```python
from build123d import *

# Parameters (mm, degrees)
SKETCH_1_R              = 4.25
EXTRUDE_1_DEPTH         = 1
SKETCH_2_R              = 3.5
EXTRUDE_2_DEPTH         = 10
HOLE_WIZARD_M31_D       = 3.4
HOLE_WIZARD_M31_DEPTH   = 5
HOLE_WIZARD_M31_TIP     = 1.021463052
CHAMFER_1_SIZE          = 0.5
HOLE_WIZARD_M31_2_D     = 2.5
HOLE_WIZARD_M31_2_DEPTH = 3
HOLE_WIZARD_M31_2_TIP   = 0.751075774


with BuildPart() as part:
    # Эскиз1 → Бобышка-Вытянуть1 (new body)
    with BuildSketch(Plane.XY):
        Circle(SKETCH_1_R)
    extrude(amount=EXTRUDE_1_DEPTH)

    # Эскиз2 → Бобышка-Вытянуть2 (add)
    with BuildSketch(Plane.XY.offset(1)):
        Circle(SKETCH_2_R)
    extrude(amount=EXTRUDE_2_DEPTH)

    # Hole Wizard M31
    with Locations(Plane.XY.offset(11)):
        with Locations((0, 0)):
            Hole(HOLE_WIZARD_M31_D / 2, depth=HOLE_WIZARD_M31_DEPTH)
            with Locations((0, 0, -(HOLE_WIZARD_M31_DEPTH + HOLE_WIZARD_M31_TIP / 2))):  # 118° drill point
                Cone(0, HOLE_WIZARD_M31_D / 2, HOLE_WIZARD_M31_TIP, mode=Mode.SUBTRACT)

    # Фаска1
    chamfer_1_edges = [part.edges().sort_by_distance(p)[0] for p in [
        (1.7, 0, 11),
    ]]
    chamfer(chamfer_1_edges, length=CHAMFER_1_SIZE)

    # Hole Wizard M31 2
    with Locations(Plane(origin=(0.206904612, 3.493879002, 8), x_dir=(0.998251143468, -0.059115603402, 0), z_dir=(0.059115603402, 0.998251143468, 0))):
        with Locations((0, 0)):
            Hole(HOLE_WIZARD_M31_2_D / 2, depth=HOLE_WIZARD_M31_2_DEPTH)
            with Locations((0, 0, -(HOLE_WIZARD_M31_2_DEPTH + HOLE_WIZARD_M31_2_TIP / 2))):  # 118° drill point
                Cone(0, HOLE_WIZARD_M31_2_D / 2, HOLE_WIZARD_M31_2_TIP, mode=Mode.SUBTRACT)


solid = part.part
```
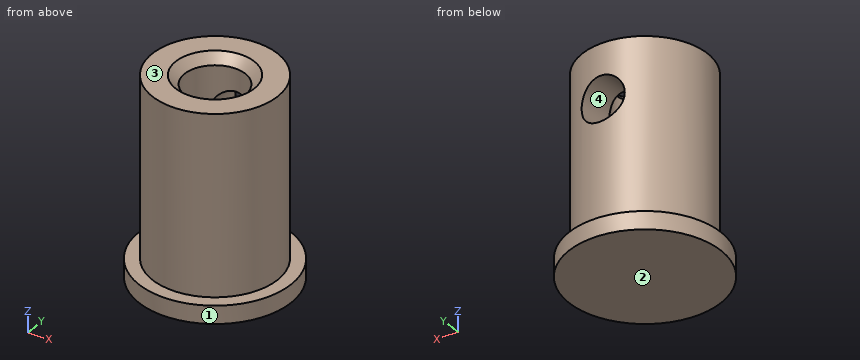
Here's how the part is built. I have some questions about the finished solid (model axes, mm). Face numbers are marked on the shaded views. Round coordinates to 2 decimals unless told otherwise and drop trailing zeros. Loops run counter-clockwise (first coordinate to the right, second up) from the corner with the lowest first, then second, coordinate; pieces in that order, holes last.
1. Will these pins go through, and if not, where does the flat tip stop? pin 1 (4 mm diameter, centred on y = 3, z = 2.5, fed in from +X); pin 2 (5 mm diameter, centred on y = 2.5, z = 9, fed in from -X).
Answers:
pin 1: stops at x = 3.91
pin 2: stops at x = -3.5
2. Suppose I cut it at C-C, the plane y = -3. Please give me the cut outline in (x, z), and give its area (3 significant figures).
Answers:
outline: (-3.01, 0) - (3.01, 0) - (3.01, 1) - (1.8, 1) - (1.8, 11) - (-1.8, 11) - (-1.8, 1) - (-3.01, 1) - close
area: 42.1 mm2
3. If I drill on probe 1 along Y at (x, z) = (0, 9.35); probe 2 along Z at (x, y) = (-4, -1); probe 3 along Y at (x, z) = (0, 8.15), over which ranges is the centre line in solid material (lowest first)?
Answers:
probe 1: y = -3.5 to -1.7, 1.7 to 3.5
probe 2: z = 0 to 1
probe 3: y = -3.5 to -1.7
4. Suppose I cut it at D-D, the plane y = 3.75. Please give me the cut outline in (x, z).
Answers:
outline: (-2, 0) - (2, 0) - (2, 1) - (-2, 1) - close
5. Thinking about a two-plate mould opening in Z: for the marked faces 1, 2, 3 and 4, which applies, released by +Z, released by -Z, zero draft, split by the parting line, or undercut?
Answers:
face 1: zero draft
face 2: released by -Z
face 3: released by +Z
face 4: undercut
6. Suppose I cut it at B-B, the plane z = 1.5. Please give me the cut outline in (x, y), and give its area (3 significant figures).
Answers:
outline: circle Ø7 at (0, 0)
area: 38.5 mm2
7. Suppose I cut it at A-A, the plane x = 3.25. Please give me the cut outline in (y, z), and give its area (3 significant figures).
Answers:
outline: (-2.74, 0) - (2.74, 0) - (2.74, 1) - (1.3, 1) - (1.3, 11) - (-1.3, 11) - (-1.3, 1) - (-2.74, 1) - close
area: 31.5 mm2
